Answer from the drawing. Dimensions are ordinates in mm from the lowest x, y and z of the part. A direction names the side the tool comes from. Give positions to 0.01 mm unless a question says otherwise; leave off trailing zeros. Write each loop counter-clockwise with the first axis right and the second up, starting at its lowest first coordinate (ties: lowest second). Pieces come first, ordered by that corner, then holes. Notation, with made-up numbers: M 89,78.5 L 138,78.5 A19 cw 138,93.5 Z; hole C 42.25,72 d8. An arc over 180 degrees is marked long. Put each result on its own line as item: value.
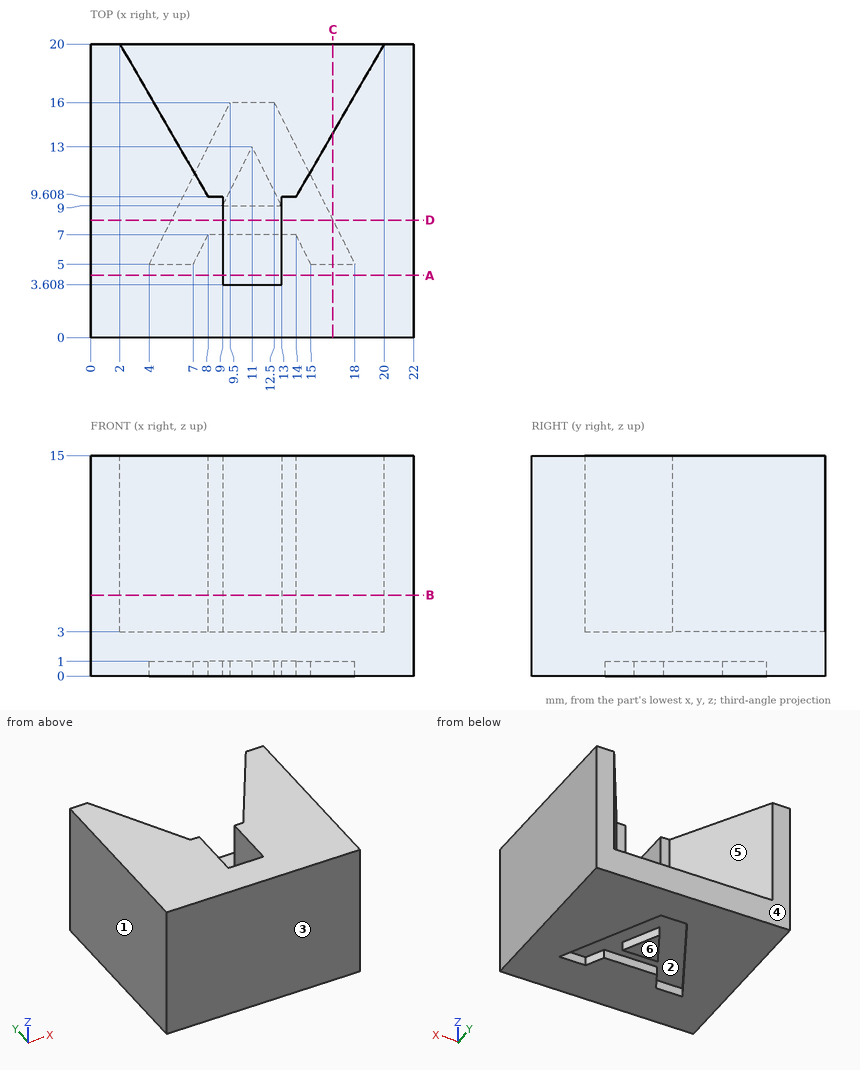
(1) For a pull along Y with two mould halves and no side action, classify the marked faces 1, 2, 3 and 4 as +Y half, -Y half, draft (parallel to the pull), parting line (faces both ways), or undercut.
Result:
face 1: draft
face 2: undercut
face 3: -Y half
face 4: +Y half
(2) Given pin 1 Ø1.1 at (x, z) = (12, 0.5) entering from -Y; pin 2 Ø0.5 at (x, z) = (13.5, 10.5) entering from +Y; pin 3 Ø1.2 at (x, z) = (11.5, 9) entering from +Y; pin 4 Ø1 at (x, z) = (15.5, 6.5) entering from +Y, each flat-ended and moving along its own axis, determine where each tip first touches the part or whether it passes through.
Result:
pin 1: stops at y = 0
pin 2: stops at y = 9.61
pin 3: stops at y = 3.61
pin 4: stops at y = 13.07
(3) Which of the six approach directions +Z, -Z, +X, -X, +Y, -Y give full straight-line access (tool end or side, diameter ignored) to the marked faces 5 and 6?
Result:
face 5: +Z, +Y
face 6: -Z, +X, -X, +Y, -Y
(4) Section C-C on x = 16.5 is taken. Determine the outline of the cut face in (y, z), and give its area (3 significant figures).
Result:
outline: M 0,0 L 5,0 L 5,1 L 8,1 L 8,0 L 20,0 L 20,3 L 13.94,3 L 13.94,15 L 0,15 Z
area: 224 mm²
(5) Section A-A on y = 4.25 is taken. Determine the outline of the cut face in (x, z), and give its area (3 significant figures).
Result:
outline: M 0,0 L 22,0 L 22,15 L 13,15 L 13,3 L 9,3 L 9,15 L 0,15 Z
area: 282 mm²
(6) Straight lines are drawn through the part: line 1 along X through (y, z) = (6.75, 12); line 2 along X through (y, z) = (12, 11.5); line 3 along Y through (x, z) = (11, 6). For each, find the intervals that lie inside material, in ascending order. Write a range as from..to.
Result:
line 1: x = 0..9, 13..22
line 2: x = 0..6.62, 15.38..22
line 3: y = 0..3.61
(7) Section D-D on y = 8 is taken. Determine the outline of the cut face in (x, z), and give its area (3 significant figures).
Result:
outline: M 0,0 L 5.5,0 L 5.5,1 L 16.5,1 L 16.5,0 L 22,0 L 22,15 L 13,15 L 13,3 L 9,3 L 9,15 L 0,15 Z
area: 271 mm²
(8) Section B-B on z = 5.5 is taken. Determine the outline of the cut face in (x, y).
Result:
outline: M 0,0 L 22,0 L 22,20 L 20,20 L 14,9.61 L 13,9.61 L 13,3.61 L 9,3.61 L 9,9.61 L 8,9.61 L 2,20 L 0,20 Z
